from build123d import *

# Parameters (mm, degrees)
F1_DEPTH = 76.2
F2_R     = 44.45
F3_DEPTH = 50.8
F4_R     = 19.05
F5_DEPTH = 50.8
F6_W     = 25.4
F6_H     = 25.4
F7_DEPTH = 25.4


with BuildPart() as f1:
    # F0 (on Front) → F1 (new body)
    with BuildSketch(Plane.XZ):
        with BuildLine():
            ThreePointArc((-49.307566, -51.592763), (-19.365586, -33.155036), (-7.651684, 0))
            ThreePointArc((-7.651684, 0), (-19.365586, 33.155036), (-49.307566, 51.592763))
            ThreePointArc((-49.307566, 51.592763), (-113.207623, 0), (-49.307566, -51.592763))
        make_face()
        with BuildLine():
            ThreePointArc((-49.307566, 51.592763), (-19.365586, 33.155036), (-7.651684, 0))
            ThreePointArc((-7.651684, 0), (-19.365586, -33.155036), (-49.307566, -51.592763))
            Line((-49.307566, -51.592763), (74.840464, -24.829606))
            ThreePointArc((74.840464, -24.829606), (44.087832, 0), (74.840464, 24.829606))
            Line((74.840464, 24.829606), (-49.307566, 51.592763))
        make_face()
        with BuildLine():
            ThreePointArc((94.887832, 0), (89.250383, 15.95624), (74.840464, 24.829606))
            ThreePointArc((74.840464, 24.829606), (44.087832, 0), (74.840464, -24.829606))
            ThreePointArc((74.840464, -24.829606), (89.250383, -15.95624), (94.887832, 0))
        make_face()
    extrude(amount=F1_DEPTH)

    # F2 (on face) → F3 (cut)
    with BuildSketch(Plane.XZ.offset(76.2)):
        with Locations((-60.429654, 0)):
            Circle(F2_R)
    extrude(amount=-F3_DEPTH, mode=Mode.SUBTRACT)

    # F4 (on face) → F5 (cut)
    with BuildSketch(Plane.XZ.offset(76.2)):
        with Locations((69.487832, 0)):
            Circle(F4_R)
    extrude(amount=-F5_DEPTH, mode=Mode.SUBTRACT)

    # F6 (on face) → F7 (join)
    with BuildSketch(Plane.XZ.offset(76.2)):
        with Locations((13.679137, 0)):
            Rectangle(F6_W, F6_H)
    extrude(amount=F7_DEPTH)


solid = f1.part
Build history of the part. All positions in model axes, mm. A direction names the side the tool comes from. Round coordinates to 2 decimals unless told otherwise and drop trailing zeros. Loops run counter-clockwise (first coordinate to the right, second up) from the corner with the lowest first, then second, coordinate; pieces in that order, holes last. Notation, with made-up numbers: (31.25, 14.5) -> (68.25, 14.5) arc R34 cw to (68.25, 49.5) -> close; hole circle Ø3 at (58, -29). An arc over 180 degrees is marked (long way). Answer in a Markdown table with one row per item.
Item 1: Mould opens along X. For faces 1 (the flat face through (69, -25.4, 0)), 2 (the flat face through (0.979, -89, 0)), 3 (the flat face through (14, -89, 12.7)), 4 (the cylindrical face through (50.456, -51.156, 0.838)) say: +X half, -X half, draft (parallel to the pull), parting line (faces both ways), or undercut.
Answers below:
| item | result |
|---|---|
| face 1 | undercut |
| face 2 | -X half |
| face 3 | draft |
| face 4 | undercut |
Item 2: Saw through at B-B (z = -10). Write the cut outline in (x, y), and give its area (3 significant figures).
Answers below:
| item | result |
|---|---|
| outline | (-112.25, -76.2) -> (-103.74, -76.2) -> (-103.74, -25.4) -> (-17.12, -25.4) -> (-17.12, -76.2) -> (0.98, -76.2) -> (0.98, -101.6) -> (26.38, -101.6) -> (26.38, -76.2) -> (53.27, -76.2) -> (53.27, -25.4) -> (85.7, -25.4) -> (85.7, -76.2) -> (92.84, -76.2) -> (92.84, 0) -> (-112.25, 0) -> close |
| area | 10,200 mm² |
Item 3: Pin check, flat tips, straight feed: pin 1 (20.5 mm diameter, centred on y = -83.5, z = 0, fed in from -X); pin 2 (1 mm diameter, centred on y = -82, z = -7, fed in from +X); pin 3 (5 mm diameter, centred on x = 50.5, y = -17.5, fed in from +Z). Stop position of each tip, or through.
Answers below:
| item | result |
|---|---|
| pin 1 | stops at x = -113.21 |
| pin 2 | stops at x = 26.38 |
| pin 3 | stops at z = 30.62 |
Item 4: Saw through at C-C (x = 61). Write the cut outline in (y, z), and give its area (3 significant figures).
Answers below:
| item | result |
|---|---|
| outline | (-76.2, -27.81) -> (0, -27.81) -> (0, 27.81) -> (-76.2, 27.81) -> (-76.2, 17.05) -> (-25.4, 17.05) -> (-25.4, -17.05) -> (-76.2, -17.05) -> close |
| area | 2,510 mm² |
Item 5: Drill centre lines: L1, parallel to X at y = -63.5, z = -1; L2, parallel to X at y = -73, z = 0.5; L3, parallel to Y at x = -37, z = 9.5. Where is each one in solid material? Low to high. Write a range as [from, to].
Answers below:
| item | result |
|---|---|
| L1 | x = [-113.2, -104.87], [-15.99, 50.46], [88.51, 94.87] |
| L2 | x = [-113.21, -104.88], [-15.98, 50.44], [88.53, 94.88] |
| L3 | y = [-25.4, 0] |
Item 6: Saw through at D-D (y = -22). Write the cut outline in (x, z).
Answers below:
| item | result |
|---|---|
| outline | (-49.31, -51.59) -> (74.84, -24.83) arc R25.4 ccw to (94.89, 0) arc R25.4 ccw to (74.84, 24.83) -> (-49.31, 51.59) arc R52.78 ccw (long way) to start |
Item 7: Which spindle directions (+Z, -Z, +X, -X, +Y, -Y) get a long thin tool onto all of the face, cutting with end or side? Do faces 5 (the flat face through (11.9, -37.6, -38.4)), 6 (the flat face through (14, -89, -12.7)), 7 (the flat face through (13.635, -37.567, 38.024)), 8 (the flat face through (-61, -25.4, 1)), 9 (the flat face through (26.379, -89, 0)). Say none if no direction does.
Answers below:
| item | result |
|---|---|
| face 5 | -Z, +X, +Y, -Y |
| face 6 | -Z, +X, -X, -Y |
| face 7 | +Z, +X, +Y, -Y |
| face 8 | -Y |
| face 9 | +Z, -Z, +X, -Y |
Item 8: Saw through at A-A (y = -55.5). Write the cut outline in (x, z).
Answers below:
| item | result |
|---|---|
| outline | (-49.31, -51.59) -> (74.84, -24.83) arc R25.4 ccw to (94.89, 0) arc R25.4 ccw to (74.84, 24.83) -> (-49.31, 51.59) arc R52.78 ccw (long way) to start; hole circle Ø88.9 at (-60.43, 0); hole circle Ø38.1 at (69.49, 0) |
